from build123d import *

# Parameters (mm, degrees)
SCHIZZO1_W                   = 120
SCHIZZO1_H                   = 82
ESTRUSIONE_ESTRUSIONE4_DEPTH = 50
SCHIZZO6_W                   = 118
SCHIZZO6_H                   = 48
TAGLIO_ESTRUSIONE2_DEPTH     = 50
SCHIZZO7_W                   = 53
SCHIZZO7_H                   = 20
ESTRUSIONE_ESTRUSIONE5_DEPTH = 27
SCHIZZO8_W                   = 52
SCHIZZO8_H                   = 19
TAGLIO_ESTRUSIONE4_DEPTH     = 27
SCHIZZO9_W                   = 5
SCHIZZO9_H                   = 1
ESTRUSIONE_ESTRUSIONE6_DEPTH = 50
SCHIZZO9_3_W                 = 113
SCHIZZO9_3_H                 = 1
ESTRUSIONE_ESTRUSIONE7_DEPTH = 1.85
SCHIZZO11_W                  = 120
SCHIZZO11_H                  = 50
SCHIZZO11_W_2                = 118
SCHIZZO11_H_2                = 48
ESTRUSIONE_ESTRUSIONE8_DEPTH = 4
SCHIZZO13_W                  = 49
SCHIZZO13_H                  = 2.3
TAGLIO_ESTRUSIONE6_DEPTH     = 119


with BuildPart() as part:
    # Schizzo1 → Estrusione-Estrusione4 (new body)
    with BuildSketch(Plane.XY):
        with Locations((60, 41)):
            Rectangle(SCHIZZO1_W, SCHIZZO1_H)
    extrude(amount=ESTRUSIONE_ESTRUSIONE4_DEPTH)

    # Schizzo6 → Taglio-Estrusione2 (cut)
    with BuildSketch(Plane.XZ):
        with Locations((60, 25)):
            Rectangle(SCHIZZO6_W, SCHIZZO6_H)
    extrude(amount=-TAGLIO_ESTRUSIONE2_DEPTH, mode=Mode.SUBTRACT)

    # Schizzo7 → Estrusione-Estrusione5 (add)
    with BuildSketch(Plane.XZ.offset(-50)):
        with Locations((27.5, 39)):
            Rectangle(SCHIZZO7_W, SCHIZZO7_H)
    extrude(amount=ESTRUSIONE_ESTRUSIONE5_DEPTH)

    # Schizzo8 → Taglio-Estrusione4 (cut)
    with BuildSketch(Plane.XZ.offset(-23)):
        with Locations((27, 39.5)):
            Rectangle(SCHIZZO8_W, SCHIZZO8_H)
    extrude(amount=-TAGLIO_ESTRUSIONE4_DEPTH, mode=Mode.SUBTRACT)

    # Schizzo9 → Estrusione-Estrusione6 (add)
    with BuildSketch(Plane(origin=(0, 50, 0), x_dir=(-1, 0, 0), z_dir=(0, -1, 0))):
        with Locations((-116.5, -4.5)):
            Rectangle(SCHIZZO9_W, SCHIZZO9_H)
    extrude(amount=ESTRUSIONE_ESTRUSIONE6_DEPTH)

    # Schizzo9<3> → Estrusione-Estrusione7 (add)
    with BuildSketch(Plane(origin=(0, 50, 0), x_dir=(-1, 0, 0), z_dir=(0, -1, 0))):
        with Locations((-57.5, -4.5)):
            Rectangle(SCHIZZO9_3_W, SCHIZZO9_3_H)
    extrude(amount=ESTRUSIONE_ESTRUSIONE7_DEPTH)

    # Schizzo11 → Estrusione-Estrusione8 (add)
    with BuildSketch(Plane.XZ):
        with Locations((60, 25)):
            Rectangle(SCHIZZO11_W, SCHIZZO11_H)
        with Locations((60, 25)):
            Rectangle(SCHIZZO11_W_2, SCHIZZO11_H_2, mode=Mode.SUBTRACT)
    extrude(amount=ESTRUSIONE_ESTRUSIONE8_DEPTH)

    # Schizzo13 → Taglio-Estrusione6 (cut)
    with BuildSketch(Plane(origin=(120, 0, 0), x_dir=(0, 0, -1), z_dir=(1, 0, 0))):
        with Locations((-25, -1.85)):
            Rectangle(SCHIZZO13_W, SCHIZZO13_H)
    extrude(amount=-TAGLIO_ESTRUSIONE6_DEPTH, mode=Mode.SUBTRACT)


solid = part.part
Could you check a few things on this model? Use its own coordinates, in mm. A direction names the side the tool comes from. Coordinates: 2 decimals unless noted, no trailing zeros. Write each loop counter-clockwise with the first axis right and the second up, starting at its lowest first coordinate (ties: lowest second). Pieces come first, ordered by that corner, then holes. Notation, with made-up numbers: (-28, -18) - (0, -18) arc R14 ccw to (0, -5) - close; hole circle Ø1 at (71.5, 50.5). An arc over 180 degrees is marked (long way). Put each result on its own line as item: value. Start each with the question number.
Q1. I want a section at B-B on y = 14. Write out the boundary of the cut face in (x, z), plus the area to 3 significant figures.
Q2. I want a section at D-D on y = 30.5. Write out the boundary of the cut face in (x, z), plus the area to 3 significant figures.
Q3. Please list where these lines run through material, in increasing order: L1, parallel to Z at x = 45, y = 40; L2, parallel to X at y = 43.5, z = 45; L3, parallel to X at y = 24, z = 22.
Q4. I want a section at C-C on x = 60. Write out the boundary of the cut face in (y, z).
Q5. Which directions (+Z, -Z, +X, -X, +Y, -Y) give clear straight access to the entire face, cutting with the end or side of a thin tool? Please do faces 1 (the flat face through (86, 49, 4)), 2 (the flat face through (59.7, -4, 49.2)).
Q6. I want a section at A-A on z = 26.5. Write out the boundary of the cut face in (x, y), plus the area to 3 significant figures.
Q7. Thinking about a two-plate mould opening in Z: for faces 3 (the flat face through (59, 40, 50)), 4 (the flat face through (59, 82, 25)), 5 (the flat face through (59, 25, 1)), which applies, pulls with the +Z half, pulls with the -Z half, needs draft (parallel to the pull), parting line crosses it, or undercut?
Q8. I'm going to push a flat-ended pin straight in: P1, Ø10, axis at x = 52.5, z = 14, coming from the -Y side. Where does the tip first touch, or does it pass through?
Checks:
1. outline: (0, 0) - (120, 0) - (120, 50) - (0, 50) - close; hole (1, 1) - (119, 1) - (119, 4) - (114, 4) - (114, 5) - (119, 5) - (119, 49) - (1, 49) - close
1. area: 341 mm²
2. outline: (0, 0) - (120, 0) - (120, 50) - (0, 50) - close; hole (1, 1) - (119, 1) - (119, 4) - (114, 4) - (114, 5) - (119, 5) - (119, 49) - (54, 49) - (54, 29) - (1, 29) - close; hole (1, 30) - (53, 30) - (53, 49) - (1, 49) - close
2. area: 413 mm²
3. L1: 0 to 1, 29 to 30, 49 to 50
3. L2: 0 to 1, 53 to 54, 119 to 120
3. L3: 0 to 1, 119 to 120
4. outline: (-4, 0) - (82, 0) - (82, 50) - (-4, 50) - (-4, 49) - (-3, 49) - (-3, 49.5) - (-0.7, 49.5) - (-0.7, 49) - (50, 49) - (50, 5) - (48.15, 5) - (48.15, 4) - (50, 4) - (50, 1) - (-0.7, 1) - (-0.7, 0.5) - (-3, 0.5) - (-3, 1) - (-4, 1) - close
5. face 1: -Y
5. face 2: +Z, -Z, +X, -X, -Y
6. outline: (0, -4) - (1, -4) - (1, 50) - (119, 50) - (119, -0.7) - (120, -0.7) - (120, 82) - (0, 82) - close; (119, -4) - (120, -4) - (120, -3) - (119, -3) - close
6. area: 3,950 mm²
7. face 3: pulls with the +Z half
7. face 4: needs draft
7. face 5: undercut
8. P1: y = 50
